```python
from build123d import *

# Parameters (mm, degrees)
SKETCH4_W           = 70.55566623
SKETCH4_H           = 46.087100556
BOSS_EXTRUDE1_DEPTH = 50


# Read off the part's stored shape, not the designer's step: AdvancedHole2
with BuildPart() as part:
    # Sketch4 → Boss-Extrude1 (new body)
    with BuildSketch(Plane.XY):
        Rectangle(SKETCH4_W, SKETCH4_H)
    extrude(amount=BOSS_EXTRUDE1_DEPTH)

    # AdvancedHole2 outline → AdvancedHole2 (revolve, cut)
    with BuildSketch(Plane.XY.offset(22.608820769)):
        Polygon((3.570986, 11.613550278), (6.746875, 11.613550278), (6.746875, 23.043550278), (0, 23.043550278), (0, -23.043550278), (2.5273, -23.043550278), (2.5273, 4.727610278), (3.356012175, 4.727610278), align=None)
    revolve(axis=Axis((0, 0, 22.608820769), (0, 1, 0)), mode=Mode.SUBTRACT)


solid = part.part
```
Design review of the part built by this model. Coordinates are the model's own, in mm. A direction names the side the tool comes from. Give positions to 0.01 mm unless a question says otherwise; leave off trailing zeros. Write each loop counter-clockwise with the first axis right and the second up, starting at its lowest first coordinate (ties: lowest second). Pieces come first, ordered by that corner, then holes.
(1) Wall thickness on line 1 along Z through (x, y) = (0, 20.25); line 2 along Z through (x, y) = (-1, 17): over which ranges is each line inside the solid? List them lowest first.
Checked values:
line 1: z = 0 to 15.86, 29.36 to 50
line 2: z = 0 to 15.94, 29.28 to 50
(2) Mouldability with a two-part tool opening along Z and no side actions: class faces 1 (the face through (0, 0, 50)), 2 (the face through (-6.74, 17.41, 22.31)), 3 (the face through (0, -23.044, 19)), 4 (the face through (-0.3, -9, 20.1)) as +Z half, -Z half, draft (parallel to the pull), parting line (faces both ways), or undercut.
Checked values:
face 1: +Z half
face 2: undercut
face 3: draft
face 4: undercut
(3) Add section A-A (x = 0). Give the boundary of the cut face in (y, z).
Checked values:
outline: (-23.04, 0) - (23.04, 0) - (23.04, 15.86) - (11.61, 15.86) - (11.61, 19.04) - (4.73, 19.25) - (4.73, 20.08) - (-23.04, 20.08) - close; (-23.04, 25.14) - (4.73, 25.14) - (4.73, 25.96) - (11.61, 26.18) - (11.61, 29.36) - (23.04, 29.36) - (23.04, 50) - (-23.04, 50) - close
(4) Clearance check with flat-ended pins moving along their axes: pin 1 Ø7.5 at (x, z) = (1.5, 24) entering from +Y; pin 2 Ø6 at (x, z) = (0, 22.61) entering from +Y. State where each tip first meets the part, or that it passes through.
Checked values:
pin 1: stops at y = 11.61
pin 2: stops at y = 4.73
(5) Tool access review of faces 5 (the face through (0, 0, 0)), 6 (the face through (-3, 11.614, 26)): name each direction out of +Z, -Z, +X, -X, +Y, -Y from which nothing blocks a thin tool from reaching the whole face with its end or side.
Checked values:
face 5: -Z, +X, -X, +Y, -Y
face 6: +Y
(6) Add section B-B (z = 17.5). Give the boundary of the cut face in (x, y).
Checked values:
outline: (-35.28, -23.04) - (35.28, -23.04) - (35.28, 23.04) - (4.41, 23.04) - (4.41, 11.61) - (-4.41, 11.61) - (-4.41, 23.04) - (-35.28, 23.04) - close
